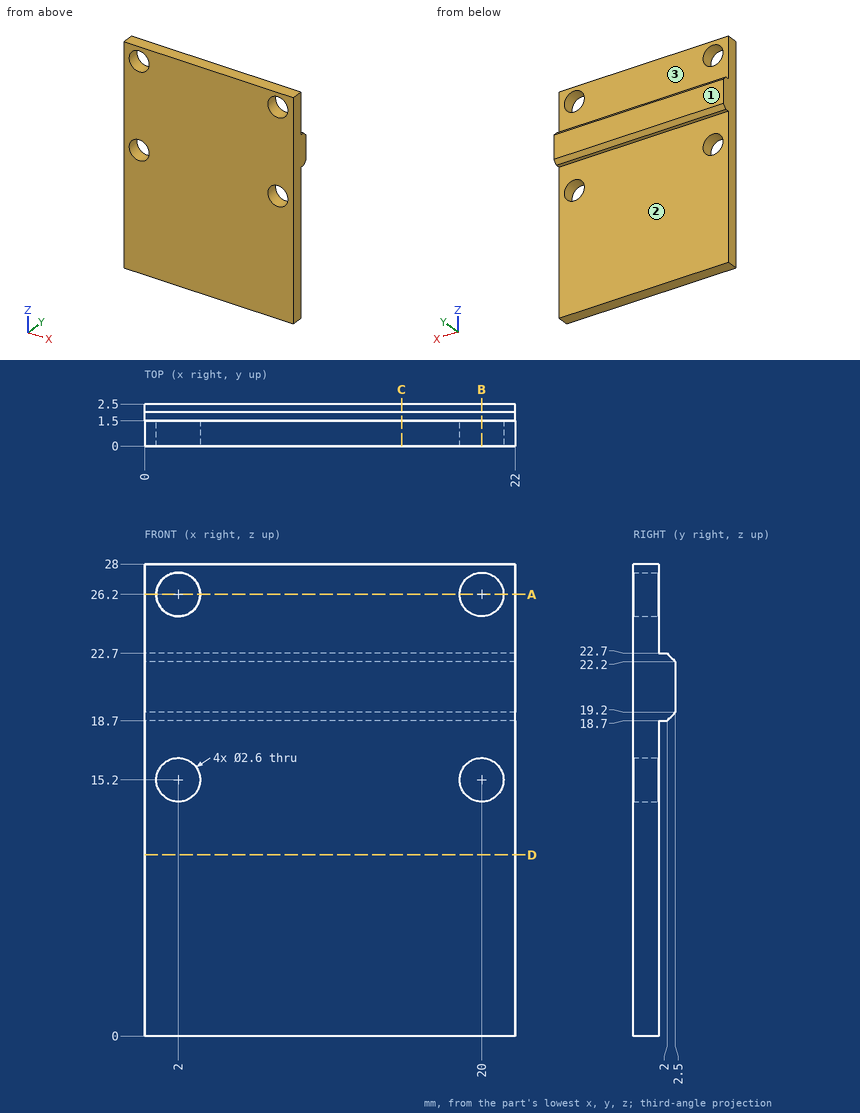
Part print with two shaded views. Sizes in mm from the minimum x, y, z corner. A direction names the side the tool comes from. Give positions to 0.01 mm unless a question says otherwise; leave off trailing zeros. Order: outer loops, then holes, each group sorted by start corner. A loop starts at its lowest first (then second) coordinate and runs counter-clockwise, first axis right, second up.
(1) Saw through at B-B, the plane x = 20. Give the cut face in (y, z).
(2) Flat gauge pins, fed straight in: pin 1 (5.5 mm diameter, centred on x = 9, z = 13, fed in from +Y); pin 2 (4 mm diameter, centred on x = 10, z = 24.5, fed in from +Y). Where does each tip first touch, or does it go through?
(3) Drill centre lines: L1, parallel to Z at x = 20, y = 0.25; L2, parallel to X at y = 1, z = 15.2; L3, parallel to Z at x = 1.25, y = 1.25. Where is each one in solid material? Low to high.
(4) Tool access for the marked faces 1, 2 and 3: list every direction of +Z, -Z, +X, -X, +Y, -Y with a clear straight run to the whole face (end or side of a thin tool).
(5) Saw through at D-D, the plane z = 10.75. Give the cut face in (x, y).
(6) Saw through at C-C, the plane x = 15.25. Give the cut face in (y, z).
(7) Saw through at A-A, the plane z = 26.2. Give the cut face in (x, y).
Results found:
1. outline: (0, 0) - (1.5, 0) - (1.5, 13.9) - (0, 13.9) - close; (0, 16.5) - (1.5, 16.5) - (1.5, 18.7) - (2, 18.7) - (2.5, 19.2) - (2.5, 22.2) - (2, 22.7) - (1.5, 22.7) - (1.5, 24.9) - (0, 24.9) - close; (0, 27.5) - (1.5, 27.5) - (1.5, 28) - (0, 28) - close
2. pin 1: stops at y = 1.5
2. pin 2: stops at y = 2.2
3. L1: z = 0 to 13.9, 16.5 to 24.9, 27.5 to 28
3. L2: x = 0 to 0.7, 3.3 to 18.7, 21.3 to 22
3. L3: z = 0 to 14.14, 16.26 to 25.14, 27.26 to 28
4. face 1: +Z, -Z, +X, -X, +Y
4. face 2: -Z, +X, -X, +Y
4. face 3: +Z, +X, -X, +Y
5. outline: (0, 0) - (22, 0) - (22, 1.5) - (0, 1.5) - close
6. outline: (0, 0) - (1.5, 0) - (1.5, 18.7) - (2, 18.7) - (2.5, 19.2) - (2.5, 22.2) - (2, 22.7) - (1.5, 22.7) - (1.5, 28) - (0, 28) - close
7. outline: (0, 0) - (0.7, 0) - (0.7, 1.5) - (0, 1.5) - close; (3.3, 0) - (18.7, 0) - (18.7, 1.5) - (3.3, 1.5) - close; (21.3, 0) - (22, 0) - (22, 1.5) - (21.3, 1.5) - close
